The listing builds one solid part. Answer for the finished solid, in the listing's coordinates (mm). A direction names the side the tool comes from. Coordinates: 2 decimals unless noted, no trailing zeros. Write each loop counter-clockwise with the first axis right and the second up, starting at its lowest first coordinate (ties: lowest second). Pieces come first, ordered by that corner, then holes.
from build123d import *

# Parameters (mm, degrees)
F1_DEPTH = 25.4
F2_W     = 25.4
F2_H     = 101.6
F3_DEPTH = 25.4
F4_R     = 8.89
F5_DEPTH = 25.4


with BuildPart() as f1:
    # F0 (on Top) → F1 (new body)
    with BuildSketch(Plane.XY):
        Polygon((25.4, -64.316225), (25.4, 37.283775), (0, 65.681839), (-25.4, 37.283775), (-25.4, -64.316225), align=None)
    extrude(amount=F1_DEPTH)

    # F2 (on face) → F3 (join)
    with BuildSketch(Plane.XY.offset(25.4)):
        with Locations((0.357762, -6.04392)):
            Rectangle(F2_W, F2_H)
    extrude(amount=F3_DEPTH)

    # F4 (on face) → F5 (join)
    with BuildSketch(Plane.XY.offset(50.8)):
        with Locations((0, -34.968402)):
            Circle(F4_R)
        with Locations((0, -2.658716)):
            Circle(F4_R)
        with Locations((0, 30.651314)):
            Circle(F4_R)
    extrude(amount=F5_DEPTH)


solid = f1.part
1. Section A-A on y = 17 is taken. Give the vertices of the cut face in (x, z).
Results found:
outline: (-25.4, 0) - (25.4, 0) - (25.4, 25.4) - (13.06, 25.4) - (13.06, 50.8) - (-12.34, 50.8) - (-12.34, 25.4) - (-25.4, 25.4) - close
2. Section B-B on z = 22 is taken. Give the vertices of the cut face in (x, y), then the cut area to 3 significant figures.
Results found:
outline: (-25.4, -64.32) - (25.4, -64.32) - (25.4, 37.28) - (0, 65.68) - (-25.4, 37.28) - close
area: 5,880 mm2
3. Section D-D on y = -9 is taken. Give the vertices of the cut face in (x, z).
Results found:
outline: (-25.4, 0) - (25.4, 0) - (25.4, 25.4) - (13.06, 25.4) - (13.06, 50.8) - (6.23, 50.8) - (6.23, 76.2) - (-6.23, 76.2) - (-6.23, 50.8) - (-12.34, 50.8) - (-12.34, 25.4) - (-25.4, 25.4) - close
4. For a pull along Y with two mould halves and no side action, classify faces 6 (the flat face through (0, 2, 0)), 7 (the flat face through (0, -56.844, 38)), 8 (the cylindrical face through (-1.157, -26.154, 63.322)) as pulls with the +Y half, pulls with the -Y half, needs draft (parallel to the pull), parting line crosses it, or undercut.
Results found:
face 6: needs draft
face 7: pulls with the -Y half
face 8: undercut
5. A tool of negligible diameter and unlimited length cuts with its end or side. For faces 1 (the flat face through (25.4, -14, 13)), 2 (the cylindrical face through (-1.927, -11.337, 63.322)), 3 (the flat face through (-12.342, -7, 38)), 4 (the flat face through (0, 44.756, 38)), 5 (the flat face through (13.058, -7, 38)), from which of +Z, -Z, +X, -X, +Y, -Y can it reach the whole face along a straight path? Write none if from no direction.
Results found:
face 1: +Z, -Z, +X, +Y, -Y
face 2: +Z
face 3: +Z, -X, +Y, -Y
face 4: +Z, +X, -X, +Y
face 5: +Z, +X, +Y, -Y
6. Section C-C on x = 11 is taken. Give the vertices of the cut face in (y, z).
Results found:
outline: (-64.32, 0) - (53.38, 0) - (53.38, 25.4) - (44.76, 25.4) - (44.76, 50.8) - (-56.84, 50.8) - (-56.84, 25.4) - (-64.32, 25.4) - close
7. Find the intervals of material crossed by L1, parallel to Y at x = 0, z = 66; L2, parallel to Y at x = 2, z = 56; L3, parallel to Z at x = 8.5, y = 43.5, in increasing order.
Results found:
L1: y = -43.86 to -26.08, -11.55 to 6.23, 21.76 to 39.54
L2: y = -43.63 to -26.31, -11.32 to 6, 21.99 to 39.31
L3: z = 0 to 50.8
8. Flat-ended cylindrical pins translate along their axes: P1, Ø2, axis at y = -7, z = 40.5, coming from the +X side; P2, Ø10, axis at x = 7.5, z = 61, coming from the -Y side; P3, Ø7.5, axis at y = 3, z = 38.5, coming from the -X side. Find the tip coordinate at first contact, or state that the pin passes through.
Results found:
P1: stops at x = 13.06
P2: stops at y = -43.5
P3: stops at x = -12.34
